The listing builds one solid part. Answer for the finished solid, in the listing's coordinates (mm). Coordinates: 2 decimals unless noted, no trailing zeros. Write each loop counter-clockwise with the first axis right and the second up, starting at its lowest first coordinate (ties: lowest second). Pieces come first, ordered by that corner, then holes. Notation, with made-up numbers: M 66,47 L 73,47 A29 ccw 73,86 Z; hole C -5.75,-4 d7. An arc over 180 degrees is marked long. Write item = value, one per line. Start each with the question number.
Autodesk Inventor part; units mm, degrees
ref_plane "YZ Plane" through (0, 0, 0) normal (1, 0, 0) x (0, 1, 0)
ref_plane "XZ Plane" through (0, 0, 0) normal (0, 1, 0) x (-1, 0, 0)
ref_plane "XY Plane" through (0, 0, 0) normal (0, 0, 1) x (1, 0, 0)
sketch "Sketch1" plane through (0, 0, 0) normal (0, 1, 0) x (-1, 0, 0)
  line L0 (0, 0) -> (-76.2, 0)
  line L1 (-76.2, 0) -> (-76.2, -50.8)
  line L2 (-76.2, -50.8) -> (0, -50.8)
  line L3 (0, -50.8) -> (0, 0)
  line L4 (0, -25.4) -> (-76.2, -25.4)
  line L5 (-38.1, -50.8) -> (-38.1, 0)
  line L6 (-6.35, -44.45) -> (-69.85, -44.45) construction
  line L7 (-69.85, -44.45) -> (-69.85, -6.35) construction
  line L8 (-69.85, -6.35) -> (-6.35, -6.35) construction
  line L9 (-6.35, -6.35) -> (-6.35, -44.45) construction
  line L10 (-6.35, -44.45) -> (-69.85, -6.35) construction
  line L11 (-69.85, -44.45) -> (-6.35, -6.35) construction
  point P0 (-38.1, -25.4)
  dimension "d0" = 76.2
  dimension "d1" = 50.8
  dimension "d2" = 63.5
  dimension "d3" = 38.1
extrude "Plate1" add sketch "Sketch1" against normal blind 2
hole "Mounting Hole" at (6.35, 0, -44.45) direction (0, -1, 0) diameter 3.81 end through all countersink diameter 7.0866 countersink angle 82
pattern_sketch "Mounting Holes" of "Mounting Hole" from (6.35, 0, -44.45) copies at (69.85, 0, -44.45) at (69.85, 0, -6.35) at (6.35, 0, -6.35)
fillet "Corner Round1" radius 3.175 4 edges at (0, -1, -50.8) (76.2, -1, -50.8) (76.2, -1, 0) (0, -1, 0)
sketch "Sketch2" plane through (0, 0, 0) normal (0, 1, 0) x (1, 0, 0)
  line L0 (5.9151, 38.1317) -> (36.83, 38.1317) construction
  line L1 (36.83, 38.1317) -> (36.83, 35.0837) construction
  line L2 (36.83, 35.0837) -> (5.9151, 35.0837) construction
  line L3 (5.9151, 35.0837) -> (5.9151, 38.1317) construction
  line L4 (5.9151, 31.2737) -> (36.83, 31.2737) construction
  line L5 (36.83, 31.2737) -> (36.83, 28.2258) construction
  line L6 (36.83, 28.2258) -> (5.9151, 28.2257) construction
  line L7 (5.9151, 28.2257) -> (5.9151, 31.2737) construction
  line L8 (11.7398, 18.288) -> (64.4602, 18.288) construction
  line L9 (64.4602, 18.288) -> (64.4602, 8.128) construction
  line L10 (64.4602, 8.128) -> (11.7398, 8.128) construction
  line L11 (11.7398, 8.128) -> (11.7398, 18.288) construction
  line L12 (21.6232, 5.588) -> (54.5768, 5.588) construction
  line L13 (54.5768, 5.588) -> (54.5768, 2.54) construction
  line L14 (54.5768, 2.54) -> (21.6232, 2.54) construction
  line L15 (21.6232, 2.54) -> (21.6232, 5.588) construction
  line L16 (5.9151, 24.4157) -> (36.83, 24.4157) construction
  line L17 (36.83, 24.4157) -> (36.83, 21.3677) construction
  line L18 (36.83, 21.3677) -> (5.9151, 21.3677) construction
  line L19 (5.9151, 21.3677) -> (5.9151, 24.4157) construction
  circle A0 centre (6.35, 6.35) radius 3.5433 construction
  circle A1 centre (69.85, 6.35) radius 3.5433 construction
  circle A2 centre (69.85, 44.45) radius 3.5433 construction
  circle A3 centre (6.35, 44.45) radius 3.5433 construction
  arc A4 (0, 3.175) -> (3.175, 0) centre (3.175, 3.175) ccw construction
  line L20 (3.175, 0) -> (73.025, 0) construction
  arc A5 (73.025, 0) -> (76.2, 3.175) centre (73.025, 3.175) ccw construction
  line L21 (76.2, 3.175) -> (76.2, 47.625) construction
  arc A6 (76.2, 47.625) -> (73.025, 50.8) centre (73.025, 47.625) ccw construction
  line L22 (73.025, 50.8) -> (3.175, 50.8) construction
  arc A7 (3.175, 50.8) -> (0, 47.625) centre (3.175, 47.625) ccw construction
  line L23 (0, 47.625) -> (0, 3.175) construction
  circle A8 centre (6.35, 44.45) radius 6.35 construction
  line L24 (73.025, 50.8) -> (3.175, 50.8)
  line L25 (38.1, 50.8) -> (38.1, 0) construction
  line L26 (0, 25.4) -> (76.2, 25.4) construction
  circle A9 centre (69.85, 44.45) radius 6.35 construction
  circle A10 centre (6.35, 6.35) radius 6.35 construction
  circle A11 centre (69.85, 6.35) radius 6.35 construction
  line L27 (39.37, 39.1478) -> (64.77, 39.1478)
  line L28 (64.77, 39.1478) -> (64.77, 34.0678)
  line L29 (64.77, 34.0678) -> (39.37, 34.0677)
  line L30 (39.37, 34.0677) -> (39.37, 39.1478)
  line L31 (39.37, 32.2897) -> (64.77, 32.2898)
  line L32 (64.77, 32.2898) -> (64.77, 27.2097)
  line L33 (64.77, 27.2097) -> (39.37, 27.2097)
  line L34 (39.37, 27.2097) -> (39.37, 32.2897)
  line L35 (39.37, 25.4317) -> (64.77, 25.4318)
  line L36 (64.77, 25.4318) -> (64.77, 20.3517)
  line L37 (64.77, 20.3517) -> (39.37, 20.3517)
  line L38 (39.37, 20.3517) -> (39.37, 25.4317)
  line L39 (13.2579, 48.26) -> (62.9421, 48.26) construction
  line L40 (62.9421, 48.26) -> (62.9421, 41.2115) construction
  line L41 (62.9421, 41.2115) -> (13.2579, 41.2115) construction
  line L42 (13.2579, 41.2115) -> (13.2579, 48.26) construction
  point P0 (38.1, 18.288)
  point P1 (38.1, 25.4)
  point P2 (38.1, 5.588)
  point P3 (38.1, 25.4)
  point P4 (39.37, 22.8917)
  point P5 (36.83, 22.8917)
  point P6 (39.37, 29.7497)
  point P7 (36.83, 29.7497)
  point P8 (39.37, 36.6077)
  point P9 (36.83, 36.6077)
  point P10 (38.1, 41.2115)
  dimension "d24" = 2.54
  dimension "d25" = 3.048
  dimension "d26" = 10.16
  dimension "d27" = 2.54
  dimension "d28" = 3.048
  dimension "d29" = 3.048
  dimension "d30" = 3.048
  dimension "d31" = 3.81
  dimension "d32" = 3.81
  dimension "d33" = 2.54
  dimension "d34" = 3.0798
  dimension "d35" = 2.54
  dimension "d36" = 25.4
  dimension "d37" = 5.08
  dimension "d38" = 7.0485
  dimension "d39" = 2.54
  dimension "d40" = 3.0798
mark "Mark1"
equation "\"d11\" = Thickness"
equation "\"d5\" = Thickness"
equation "\"largeTextHeight\" = 3.048"
equation "\"smallTextHeight\" = 2.54"
properties part number "Jack Plate" material "Aluminum 6061"
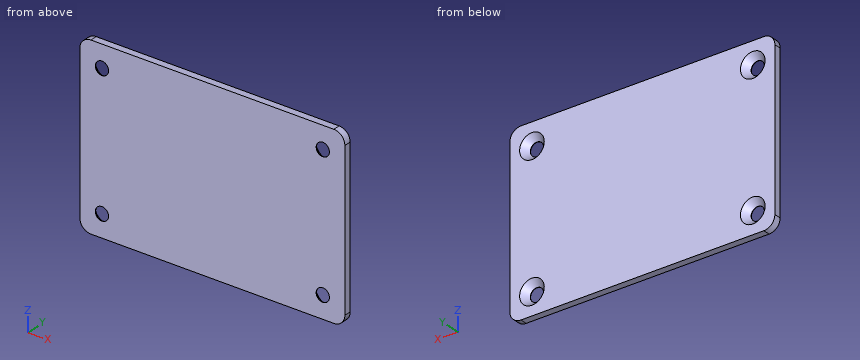
1. Straight lines are drawn through the part: L1, parallel to X at y = -1.9, z = -44.45 (3 decimals); L2, parallel to Z at x = 69.85, y = -1.95 (3 decimals); L3, parallel to X at y = -1.3, z = -46. For each, find the intervals that lie inside material, in ascending order. Write a range as [from, to].
2. The part is cut by section B-B, the plane z = -6.35. Write down the section's boundary in (x, y) (3 decimals).
3. The part is cut by section C-C, the plane y = -0.65. Write down the section's boundary in (x, z) (3 decimals), and give its area (3 significant figures).
4. Each of these flat-tipped pins is pushed along its axis until it touches: pin 1 (4.5 mm diameter, centred on x = 69.85, z = -6.35, fed in from +Y); pin 2 (12 mm diameter, centred on x = 44.5, z = -19.5, fed in from +Y); pin 3 (6 mm diameter, centred on x = 6.35, z = -44.45, fed in from +Y) (3 decimals). Where does it stop, or does it pass through?
5. The part is cut by section A-A, the plane x = 69.85. Write down the section's boundary in (y, z) (3 decimals), and give its area (3 significant figures).
Solution:
q1.L1 = [0, 4.445], [8.255, 67.945], [71.755, 76.2]
q1.L2 = [-50.8, -46.355], [-42.545, -8.255], [-4.445, 0]
q1.L3 = [0, 4.5], [8.2, 68], [71.7, 76.2]
q2.outline = M 0,-2 L 4.445,-2 L 4.445,-1.885 L 2.807,0 L 0,0 Z; M 8.255,-2 L 67.945,-2 L 67.945,-1.885 L 66.307,0 L 9.893,0 L 8.255,-1.885 Z; M 71.755,-2 L 76.2,-2 L 76.2,0 L 73.393,0 L 71.755,-1.885 Z
q3.outline = M 0,-47.625 A3.175 ccw 3.175,-50.8 L 73.025,-50.8 A3.175 ccw 76.2,-47.625 L 76.2,-3.175 A3.175 ccw 73.025,0 L 3.175,0 A3.175 ccw 0,-3.175 Z; hole C 6.35,-44.45 d5.957; hole C 6.35,-6.35 d5.957; hole C 69.85,-44.45 d5.957; hole C 69.85,-6.35 d5.957
q3.area = 3,750 mm^2
q4.pin_1 = -1.49
q4.pin_2 = 0
q4.pin_3 = -0.625
q5.outline = M -2,-50.8 L 0,-50.8 L 0,-47.993 L -1.885,-46.355 L -2,-46.355 Z; M -2,-42.545 L -1.885,-42.545 L 0,-40.907 L 0,-9.893 L -1.885,-8.255 L -2,-8.255 Z; M -2,-4.445 L -1.885,-4.445 L 0,-2.807 L 0,0 L -2,0 Z
q5.area = 80.2 mm^2
